Design review of the part built by this model. Coordinates are the model's own, in mm. A direction names the side the tool comes from. Give positions to 0.01 mm unless a question says otherwise; leave off trailing zeros. Write each loop counter-clockwise with the first axis right and the second up, starting at its lowest first coordinate (ties: lowest second). Pieces come first, ordered by that corner, then holes. Notation, with made-up numbers: (50, -36) -> (87, -36) arc R37 cw to (87, 1) -> close; hole circle Ø8 at (54, 54). An arc over 180 degrees is marked (long way). Use CSV: the item, a comma, the result in double quotes.
```python
from build123d import *

# Parameters (mm, degrees)
PAD_DEPTH    = 8
CHAMFER_SIZE = 1.5


with BuildPart() as part:
    # Sketch → Pad (new body)
    with BuildSketch(Plane.XY):
        with BuildLine():
            ThreePointArc((31.65, 0), (46.706124, 22.957835), (19.65001, 27.617855))
            ThreePointArc((19.65001, 27.617855), (19.832321, 22.317689), (25.132488, 22.5))
            ThreePointArc((31.65, 7.5), (39.827391, 19.969016), (25.132488, 22.5))
            Line((31.65, 7.5), (19.65001, 7.5))
            Line((19.65001, 7.5), (0, 0))
            Line((0, 0), (0, -40))
            Line((0, -40), (6, -40))
            Line((6, -40), (6, -5))
            Line((6, -5), (25.65, -5))
            Line((25.65, -5), (25.65, -40))
            Line((25.65, -40), (31.65, -40))
            Line((31.65, -40), (31.65, 0))
        make_face()
    extrude(amount=PAD_DEPTH)

    # Chamfer
    chamfer_edges = [part.edges().sort_by_distance(p)[0] for p in [
        (6, -40, 4),
        (25.65, -40, 4),
    ]]
    chamfer(chamfer_edges, length=CHAMFER_SIZE)


solid = part.part
```
(1) Tool access review of faces 1 (the face through (6, -22, 4)), 2 (the face through (31.65, -20, 4)), 3 (the face through (24, -1, 0)): name each direction out of +Z, -Z, +X, -X, +Y, -Y from which nothing blocks a thin tool from reaching the whole face with its end or side.
Established:
face 1,"+Z, -Z, -Y"
face 2,"+Z, -Z, +X, -Y"
face 3,"-Z, +X, -X, +Y, -Y"
(2) Take a section at D-D (y = -1). Write out the cut boundary in (x, z), then the cut area to 3 significant figures.
Established:
outline,"(0, 0) -> (31.65, 0) -> (31.65, 8) -> (0, 8) -> close"
area,"253 mm2"
(3) For line 1 along X through (y, z) = (-13, 1); line 2 along Y through (x, z) = (28, 3.5); line 3 along X through (y, z) = (-2, 3.5), list the stretches that pass through material, from the lowest coordinate up. Write a range as [from, to].
Established:
line 1,"x = [0, 6], [25.65, 31.65]"
line 2,"y = [-40, 7.5], [24.55, 32.42]"
line 3,"x = [0, 31.65]"
(4) Take a section at C-C (z = 1.5). Write out the cut boundary in (x, y).
Established:
outline,"(0, -40) -> (4.5, -40) -> (6, -38.5) -> (6, -5) -> (25.65, -5) -> (25.65, -38.5) -> (27.15, -40) -> (31.65, -40) -> (31.65, 0) arc R16.42 ccw (long way) to (19.65, 27.62) arc R3.75 ccw to (25.13, 22.5) arc R8.92 cw (long way) to (31.65, 7.5) -> (19.65, 7.5) -> (0, 0) -> close"
(5) Mouldability with a two-part tool opening along Y and no side actions: class faces 4 (the face through (26, 7.5, 4)), 5 (the face through (25.65, -22, 4)), 6 (the face through (39.923, 19.741, 3.944)), 7 (the face through (26.41, -39.26, 3.94)) as +Y half, -Y half, draft (parallel to the pull), parting line (faces both ways), or undercut.
Established:
face 4,"undercut"
face 5,"draft"
face 6,"undercut"
face 7,"-Y half"
(6) Take a section at B-B (x = 30). Write out the cut boundary in (y, z).
Established:
outline,"(-40, 0) -> (7.5, 0) -> (7.5, 8) -> (-40, 8) -> close; (25.18, 0) -> (32.75, 0) -> (32.75, 8) -> (25.18, 8) -> close"
(7) Clearance check with flat-ended pins moving along their axes: pin 1 (3 mm diameter, centred on x = 12.5, z = 5.5, fed in from -Y); pin 2 (16 mm diameter, centred on x = 31.65, y = 16.42, fed in from +Z). State where each tip first meets the part, or that it passes through.
Established:
pin 1,"stops at y = -5"
pin 2,"passes through"
(8) Take a section at A-A (y = -29.5). Write out the cut boundary in (x, z).
Established:
outline,"(0, 0) -> (6, 0) -> (6, 8) -> (0, 8) -> close; (25.65, 0) -> (31.65, 0) -> (31.65, 8) -> (25.65, 8) -> close"
